Can you work these out from the model? Positions are in its coordinate system, mm. Face numbers are marked on the shaded views. A direction names the side the tool comes from. Round coordinates to 2 decimals unless told otherwise and drop trailing zeros. Write each loop counter-clockwise with the first axis right and the second up, starting at its lowest first coordinate (ties: lowest second). Pieces come first, ordered by that corner, then holes.
Q1. If we section it at C-C (x = 68): Please give me the cut outline in (y, z) (3 decimals).
Q2. If we section it at B-B (x = 44.5): Please give me the cut outline in (y, z), plus the area to 3 significant figures.
Q3. I'm going to push flat-ended pins straight in: pin 1 Ø10.5 at (y, z) = (-2.5, 13.5) entering from +X; pin 2 Ø5 at (x, y) = (22, 6.5) entering from -Z; pin 3 Ø6.5 at (x, y) = (68.5, 13) entering from +Z (3 decimals). Where does each tip first touch, or does it pass through?
Q4. For the marked faces 1, 2, 3 and 4, which set-ups out of +Z, -Z, +X, -X, +Y, -Y let a thin tool reach every point of the face, with its end or its side?
Q5. If we section it at A-A (y = 0): Please give me the cut outline in (x, z), plus the area to 3 significant figures.
Q6. We'd pull the mould along X, two halves only. Please class the marked faces 5, 6 and 7: +X half, -X half, draft (parallel to the pull), parting line (faces both ways), or undercut.
Q7. If we section it at D-D (y = 21): Please give me the cut outline in (x, z) (3 decimals).
Q8. Please list where these lines run through material, in increasing order: line 1 along Z through (x, y) = (25, 0); line 2 along X through (y, z) = (15.5, -4).
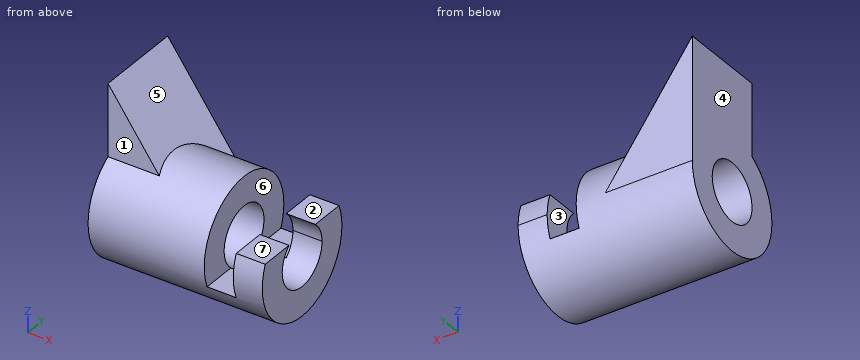
from build123d import *

# Parameters (mm, degrees)
F0_R          = 12.7
F1_DEPTH      = 76.2
F3_DEPTH      = 25.401
F3_DEPTH_BACK = 25.4
F5_DEPTH      = 25.4
F6_DEPTH      = 12.7
F7_DEPTH      = 50.8


with BuildPart() as f1:
    # F0 (on Right) → F1 (new body)
    with BuildSketch(Plane.YZ):
        with BuildLine():
            ThreePointArc((-19.5864308625, 16.171942557), (-8.5925740058, -23.9024616296), (25.4, 0))
            ThreePointArc((25.4, 0), (8.5925740058, 23.9024616296), (-19.5864308625, 16.171942557))
        make_face()
        Circle(F0_R, mode=Mode.SUBTRACT)
    extrude(amount=F1_DEPTH)

    # F2 (on Front) → F3 (cut, two sides)
    with BuildSketch(Plane.XZ) as f3_sk:
        Polygon((76.2, 9.525), (76.2, 25.4), (50.8, 25.4), (50.8, -9.525), (63.5, -9.525), (63.5, 9.525), align=None)
    extrude(amount=-F3_DEPTH, mode=Mode.SUBTRACT)
    extrude(f3_sk.sketch, amount=F3_DEPTH_BACK, mode=Mode.SUBTRACT)

    # F4 (on Front) → F5 (join)
    with BuildSketch(Plane.XZ):
        Polygon((38.1, 0), (0, 53.5043813288), (0, 0), align=None)
    extrude(amount=-F5_DEPTH)

    # F4 (on Front) → F6 (join)
    with BuildSketch(Plane.XZ):
        Polygon((38.1, 0), (0, 53.5043813288), (0, 0), align=None)
    extrude(amount=F6_DEPTH)

    # F0 (on Right) → F7 (cut)
    with BuildSketch(Plane.YZ):
        Circle(F0_R)
    extrude(amount=F7_DEPTH, mode=Mode.SUBTRACT)


solid = f1.part
A:
1. outline: (-23.546, 9.525) arc R25.4 ccw (long way) to (23.546, 9.525) - (8.4, 9.525) arc R12.7 cw (long way) to (-8.4, 9.525) - close
2. outline: circle Ø50.8 at (0, 0); hole circle Ø25.4 at (0, 0)
2. area: 1,520 mm2
3. pin 1: stops at x = 50.8
3. pin 2: stops at z = -25.08
3. pin 3: stops at z = 9.525
4. face 1: +Z, +X, -X, -Y
4. face 2: +Z, +X, +Y, -Y
4. face 3: +Z, +Y, -Y
4. face 4: +Z, -Z, -X, +Y, -Y
5. outline: (0, -25.4) - (76.2, -25.4) - (76.2, -12.7) - (0, -12.7) - close; (0, 12.7) - (50.8, 12.7) - (50.8, 25.4) - (20.01, 25.4) - (0, 53.5) - close
5. area: 1,890 mm2
6. face 5: +X half
6. face 6: undercut
6. face 7: draft
7. outline: (0, -14.288) - (76.2, -14.288) - (76.2, 9.525) - (63.5, 9.525) - (63.5, -9.525) - (50.8, -9.525) - (50.8, 14.288) - (27.925, 14.288) - (0, 53.504) - close
8. line 1: z = -25.4 to -12.7, 12.7 to 25.4
8. line 2: x = 0 to 50.8, 63.5 to 76.2
